Autodesk Inventor part; units mm, degrees
ref_plane "YZ Plane" through (0, 0, 0) normal (1, 0, 0) x (0, 1, 0)
ref_plane "XZ Plane" through (0, 0, 0) normal (0, 1, 0) x (-1, 0, 0)
ref_plane "XY Plane" through (0, 0, 0) normal (0, 0, 1) x (1, 0, 0)
sketch "スケッチ1" plane through (0, 0, 0) normal (0, 0, 1) x (1, 0, 0)
  line L0 (-33, 22.7) -> (33, 22.7)
  line L1 (33, 22.7) -> (33, 0)
  line L2 (33, 0) -> (-33, 0)
  line L3 (-33, 0) -> (-33, 22.7)
  point P0 (0, 0)
  point P1 (0, 0)
  dimension "d0" = 66
  dimension "d1" = 22.7
extrude "押し出し1" add sketch "スケッチ1" along normal blind 2
sketch "スケッチ3" plane through (0, 0, 0) normal (0, 0, -1) x (-1, 0, 0)
  line L0 (-7.5, 4) -> (7.5, 4)
  line L1 (7.5, 4) -> (7.5, -7.5)
  line L2 (7.5, -7.5) -> (-7.5, -7.5)
  line L3 (-7.5, -7.5) -> (-7.5, 4)
  line L4 (33, 0) -> (-33, 0)
  point P0 (0, 0)
  point P1 (0, 4)
  point P2 (0, 0)
  dimension "d4" = 15
  dimension "d5" = 11.5
  dimension "d6" = 4
extrude "押し出し2" add sketch "スケッチ3" along normal blind 1.6
sketch "スケッチ4" plane through (0, 0, -1.6) normal (0, 0, -1) x (-1, 0, 0)
  line L0 (-5.08, -3.81) -> (5.08, -3.81)
  line L1 (5.08, -3.81) -> (5.08, -6.35)
  line L2 (5.08, -6.35) -> (-5.08, -6.35)
  line L3 (-5.08, -6.35) -> (-5.08, -3.81)
  point P0 (0, 0)
  point P1 (0, -3.81)
  point P2 (5.08, -5.08)
  dimension "d9" = 10.16
  dimension "d10" = 2.54
  dimension "d11" = 5.08
extrude "押し出し3" add sketch "スケッチ4" along normal blind 11
properties part number "AE-AQM1602A"
Verification items for the finished model (mm, model axes). A direction names the side the tool comes from. Coordinates: 2 decimals unless noted, no trailing zeros. Loops run counter-clockwise (first coordinate to the right, second up) from the corner with the lowest first, then second, coordinate; pieces in that order, holes last. Notation, with made-up numbers: (66, 39.25) - (90, 39.25) arc R12 ccw to (90, 57.25) - close; hole circle Ø2 at (36, 86.25). An arc over 180 degrees is marked (long way). Return JSON: item names as keys, results as strings.
1. Section check A-A, the plane y = 1. Record the boundary of the cut face in (x, z), then the cut area to 3 significant figures.
Established:
{"outline": "(-33, 0) - (-7.5, 0) - (-7.5, -1.6) - (7.5, -1.6) - (7.5, 0) - (33, 0) - (33, 2) - (-33, 2) - close", "area": "156 mm2"}
2. Tool access check on faces 1 (the flat face through (0, -6.35, -7)), 2 (the flat face through (-5.08, -5, -7)), 3 (the flat face through (0, -4, 0)), 4 (the flat face through (0, -3.81, -7)). Record the directions out of +Z, -Z, +X, -X, +Y, -Y that give a thin tool (end or side, any length) a straight path to the whole face; none if there is none.
Established:
{"face 1": "-Z, +X, -X, -Y", "face 2": "-Z, -X, +Y, -Y", "face 3": "+Z, +X, -X, -Y", "face 4": "-Z, +X, -X, +Y"}
3. Go/stop test with flat-tipped pins: pin 1 (8 mm diameter, centred on x = 0.5, z = -7.5, fed in from +Y); pin 2 (1 mm diameter, centred on x = -2, z = 1, fed in from -Y); pin 3 (1.5 mm diameter, centred on x = -24, z = -1, fed in from -Y); pin 4 (11.5 mm diameter, centred on x = 3, y = 12.5, fed in from -Z). Record where each tip stops, or that it passes through.
Established:
{"pin 1": "stops at y = -3.81", "pin 2": "stops at y = 0", "pin 3": "passes through", "pin 4": "stops at z = 0"}
4. Section check C-C, the plane z = -0.75. Record the boundary of the cut face in (x, y), then the cut area to 4 significant figures.
Established:
{"outline": "(-7.5, -7.5) - (7.5, -7.5) - (7.5, 4) - (-7.5, 4) - close", "area": "172.5 mm2"}
5. Thickness scan on L1, parallel to Z at x = -22.5, y = 3; L2, parallel to Y at x = -20.5, z = 0.5; L3, parallel to X at y = -4.5, z = -3.25. Record the ranges inside material, lowest first.
Established:
{"L1": "z = 0 to 2", "L2": "y = 0 to 22.7", "L3": "x = -5.08 to 5.08"}
6. Section check B-B, the plane x = -0.5. Record the boundary of the cut face in (y, z), then the cut area to 3 significant figures.
Established:
{"outline": "(-7.5, -1.6) - (-6.35, -1.6) - (-6.35, -12.6) - (-3.81, -12.6) - (-3.81, -1.6) - (4, -1.6) - (4, 0) - (22.7, 0) - (22.7, 2) - (0, 2) - (0, 0) - (-7.5, 0) - close", "area": "91.7 mm2"}
7. Section check D-D, the plane x = -22.5. Record the boundary of the cut face in (y, z), then the cut area to 3 significant figures.
Established:
{"outline": "(0, 0) - (22.7, 0) - (22.7, 2) - (0, 2) - close", "area": "45.4 mm2"}
8. Mould release check, pull along Z, two halves, no side actions. Record for faces 5 (the flat face through (-7.5, -2, -1)), 6 (the flat face through (0, 12, 2)), 7 (the flat face through (0, -5, -12.6)): +Z half, -Z half, draft (parallel to the pull), parting line (faces both ways), or undercut.
Established:
{"face 5": "draft", "face 6": "+Z half", "face 7": "-Z half"}
